Can you work these out from the model? Positions are in its coordinate system, mm. A direction names the side the tool comes from. Round coordinates to 2 decimals unless told otherwise and drop trailing zeros. Loops run counter-clockwise (first coordinate to the right, second up) from the corner with the lowest first, then second, coordinate; pieces in that order, holes last.
```python
from build123d import *

# Parameters (mm, degrees)
SKETCH1_R           = 2
SKETCH1_R_2         = 8
SKETCH1_R_3         = 1.5
BOSS_EXTRUDE1_DEPTH = 7


with BuildPart() as part:
    # Sketch1 → Boss-Extrude1 (new, symmetric)
    with BuildSketch(Plane.XY):
        with BuildLine():
            Line((-50, 9), (50, 9))
            ThreePointArc((50, 9), (59, 0), (50, -9))
            Line((50, -9), (-50, -9))
            ThreePointArc((-50, -9), (-59, 0), (-50, 9))
        make_face()
        with Locations((-30, 0)):
            Circle(SKETCH1_R, mode=Mode.SUBTRACT)
        with Locations((30, 0)):
            Circle(SKETCH1_R, mode=Mode.SUBTRACT)
        with Locations((-50, 0)):
            Circle(SKETCH1_R_2, mode=Mode.SUBTRACT)
        with Locations((50, 0)):
            Circle(SKETCH1_R_2, mode=Mode.SUBTRACT)
        with Locations((20, -5)):
            Circle(SKETCH1_R_3, mode=Mode.SUBTRACT)
        with Locations((20, 5)):
            Circle(SKETCH1_R_3, mode=Mode.SUBTRACT)
        with BuildLine():
            Line((-12, -2.5), (-12, 2.5))
            ThreePointArc((-12, 2.5), (-10, 4.5), (-8, 2.5))
            Line((-8, 2.5), (-8, -2.5))
            ThreePointArc((-8, -2.5), (-10, -4.5), (-12, -2.5))
        make_face(mode=Mode.SUBTRACT)
        with BuildLine():
            Line((12, -2.5), (12, 2.5))
            ThreePointArc((12, 2.5), (10, 4.5), (8, 2.5))
            Line((8, 2.5), (8, -2.5))
            ThreePointArc((8, -2.5), (10, -4.5), (12, -2.5))
        make_face(mode=Mode.SUBTRACT)
    extrude(amount=BOSS_EXTRUDE1_DEPTH, both=True)


solid = part.part
```
(1) If I drill on line 1 (Y direction, x = 20, z = 1.25); line 2 (X direction, y = 6.25, z = 0.5); line 3 (X direction, y = -2.5, z = -5), over which ranges is the centre line in solid material (lowest first)?
(2) For pin 1 (5.5 mm diameter, centred on y = 0.5, z = 3.5, fed in from -X); pin 2 (1.8 mm diameter, centred on x = 20, y = -5, fed in from +Z); pin 3 (2 mm diameter, centred on y = 4.5, z = 1.5, fed in from +X); pin 4 (1 mm diameter, centred on y = 3.5, z = 1.5, fed in from -X), each with a flat end and sliding along its axis, tell me the tip position at first contact or that it passes through.
(3) Which directions (+Z, -Z, +X, -X, +Y, -Y) give clear straight access to the entire face, cutting with the end or side of a thin tool? Please do faces 5 (the cylindrical face through (10, 4.5, 0.1)), 6 (the flat face through (1, -9, 0)).
(4) Suppose I cut it at D-D (x = -30). Write out the boundary of the cut face in (y, z).
(5) We'd pull the mould along Y, two halves only. Please class faces 1 (the flat face through (-1, 9, 0)), 2 (the cylindrical face through (18.5, -4.93, -0.1)), 3 (the flat face through (1, 0, -7)), 4 (the flat face through (-8, 0, 0)): released by +Y, released by -Y, zero draft, split by the parting line, or undercut.
(6) Suppose I cut it at B-B (y = 0). Write out the boundary of the cut face in (x, z).
(7) Suppose I cut it at A-A (x = 20). Write out the boundary of the cut face in (y, z), then the cut area to 3 significant figures.
(8) Suppose I cut it at C-C (z = 0.75). Give the number of separate pieces and of enclosed holes in the cut face, then the cut area to 3 significant figures.
Check result:
1. line 1: y = -9 to -6.5, -3.5 to 3.5, 6.5 to 9
1. line 2: x = -56.48 to -54.99, -45.01 to 19.17, 20.83 to 45.01, 54.99 to 56.48
1. line 3: x = -58.65 to -57.6, -42.4 to -12, -8 to 8, 12 to 42.4, 57.6 to 58.65
2. pin 1: stops at x = -59
2. pin 2: passes through
2. pin 3: stops at x = 58.29
2. pin 4: stops at x = -58.49
3. face 5: +Z, -Z
3. face 6: +Z, -Z, +X, -X, -Y
4. outline: (-9, -7) - (-2, -7) - (-2, 7) - (-9, 7) - close; (2, -7) - (9, -7) - (9, 7) - (2, 7) - close
5. face 1: released by +Y
5. face 2: undercut
5. face 3: zero draft
5. face 4: undercut
6. outline: (-59, -7) - (-58, -7) - (-58, 7) - (-59, 7) - close; (-42, -7) - (-32, -7) - (-32, 7) - (-42, 7) - close; (-28, -7) - (-12, -7) - (-12, 7) - (-28, 7) - close; (-8, -7) - (8, -7) - (8, 7) - (-8, 7) - close; (12, -7) - (28, -7) - (28, 7) - (12, 7) - close; (32, -7) - (42, -7) - (42, 7) - (32, 7) - close; (58, -7) - (59, -7) - (59, 7) - (58, 7) - close
7. outline: (-9, -7) - (-6.5, -7) - (-6.5, 7) - (-9, 7) - close; (-3.5, -7) - (3.5, -7) - (3.5, 7) - (-3.5, 7) - close; (6.5, -7) - (9, -7) - (9, 7) - (6.5, 7) - close
7. area: 168 mm2
8. separate pieces: 1
8. enclosed holes: 8
8. area: 1,550 mm2
